Autodesk Inventor part; units mm, degrees
ref_plane "YZ Plane" through (0, 0, 0) normal (1, 0, 0) x (0, 1, 0)
ref_plane "XZ Plane" through (0, 0, 0) normal (0, 1, 0) x (-1, 0, 0)
ref_plane "XY Plane" through (0, 0, 0) normal (0, 0, 1) x (1, 0, 0)
sketch "Sketch1" plane through (0, 0, 0) normal (0, 1, 0) x (-1, 0, 0)
  line L0 (275, 225) -> (-275, 225)
  line L1 (-275, 225) -> (-275, -225)
  line L2 (-275, -225) -> (275, -225)
  line L3 (275, -225) -> (275, 225)
  line L4 (275, 225) -> (-275, -225) construction
  line L5 (-275, 225) -> (275, -225) construction
  point P0 (0, 0)
  dimension "d0" = 550
  dimension "d1" = 450
extrude "Extrusion1" add sketch "Sketch1" against normal blind 15
sketch "Sketch2" plane through (0, -15, 0) normal (0, -1, 0) x (1, 0, 0)
  line L0 (275, -225) -> (275, 225)
  line L1 (275, 225) -> (225, 225)
  line L2 (225, 225) -> (225, 175)
  line L3 (225, 175) -> (275, 175)
  line L4 (275, 175) -> (275, 225)
  line L5 (-275, -225) -> (275, -225)
  line L6 (275, -225) -> (225, -225)
  line L7 (225, -225) -> (225, -175)
  line L8 (225, -175) -> (275, -175)
  line L9 (275, -175) -> (275, -225)
  line L10 (-275, 225) -> (-275, -225)
  line L11 (-275, -225) -> (-225, -225)
  line L12 (-225, -225) -> (-225, -175)
  line L13 (-225, -175) -> (-275, -175)
  line L14 (-275, -175) -> (-275, -225)
  line L15 (-275, 225) -> (-225, 225)
  line L16 (-225, 225) -> (-225, 175)
  line L17 (-225, 175) -> (-275, 175)
  line L18 (-275, 175) -> (-275, 225)
  point P0 (0, 0)
  dimension "d4" = 50
  dimension "d5" = 50
  dimension "d6" = 50
  dimension "d7" = 50
extrude "Extrusion2" add sketch "Sketch2" along normal blind 500
sketch "Sketch3" plane through (0, -515, 0) normal (0, -1, 0) x (1, 0, 0)
  line L0 (225, 175) -> (275, 175)
  line L1 (225, 175) -> (265, 175)
  line L2 (265, 175) -> (265, 215)
  line L3 (265, 215) -> (225, 215)
  line L4 (225, 215) -> (225, 175)
  point P0 (0, 0)
  dimension "d10" = 40
  dimension "d11" = 40
extrude "Extrusion3" cut sketch "Sketch3" against normal blind 500
mirror "Mirror1" about plane through (0, 0, 0) normal (1, 0, 0) of "Extrusion3"
mirror "Mirror2" about plane through (0, 0, 0) normal (0, 0, 1) of "Extrusion3"
sketch "Sketch4" plane through (0, -515, 0) normal (0, -1, 0) x (1, 0, 0)
  line L0 (-275, -175) -> (-225, -175)
  line L1 (-225, -175) -> (-265, -175)
  line L2 (-265, -175) -> (-265, -215)
  line L3 (-265, -215) -> (-225, -215)
  line L4 (-225, -215) -> (-225, -175)
  point P0 (0, 0)
  dimension "d14" = 40
  dimension "d15" = 40
extrude "Extrusion4" cut sketch "Sketch4" against normal blind 500
sketch "Sketch5" plane through (0, 0, 0) normal (0, 1, 0) x (1, 0, 0)
  line L0 (275, -225) -> (275, 225)
  line L1 (275, 0) -> (265, 0)
  line L2 (265, 0) -> (265, -19.5)
  line L3 (265, -19.5) -> (265, 9.5)
  circle A0 centre (265, 9.5) radius 2.5
  circle A1 centre (265, -19.5) radius 2.5
  point P0 (0, 0)
  dimension "d18" = 10
  dimension "d19" = 19.5
  dimension "d20" = 29
  dimension "d21" = 5
  dimension "d22" = 5
extrude "Extrusion5" cut sketch "Sketch5" against normal through all
thread "Thread1"
thread "Thread2"
ref_plane "Work Plane1" through (0, 0, 0) normal (1, 0, 0) x (0, 1, 0)
ref_plane "Work Plane2" through (0, 0, 0) normal (0, 0, 1) x (1, 0, 0)
properties part number "Work table" material "Steel, Mild"
CAD build for the part. Positions are in the model's coordinates, mm. A direction names the side the tool comes from. Round coordinates to 2 decimals unless told otherwise and drop trailing zeros. Order: outer loops, then holes, each group sorted by start corner. A loop starts at its lowest first (then second) coordinate and runs counter-clockwise, first axis right, second up. Notation, with made-up numbers: (86.5, 2.25) -> (104.5, 2.25) arc R26 cw to (104.5, 38.25) -> close; hole circle Ø5 at (-19, 34.5). An arc over 180 degrees is marked (long way). Write item = value, one per line. Start each with the question number.
(1) Pin check, flat tip, straight feed: P1, Ø12, axis at x = 158.5, z = -90, coming from the +Y side. Stop position of the tip, or through.
(2) Cut at C-C, the plane z = 62. List the corners of the cut face in (x, y), then the cut area to 3 significant figures.
(3) Cut at B-B, the plane x = -238.5. List the corners of the cut face in (y, z), then the cut area to 4 significant figures.
(4) Which spindle directions (+Z, -Z, +X, -X, +Y, -Y) get a long thin tool onto all of the face, cutting with end or side? Do faces 4 (the flat face through (265, -268, -195)), 5 (the flat face through (-225.4, -237.2, 225)). Say none if no direction does.
(5) Cut at D-D, the plane x = 169.5. List the corners of the cut face in (y, z), then the cut area to 3 significant figures.
(6) Cut at A-A, the plane y = -128. List the corners of the cut face in (x, z).
(7) Probe line 1 (Z direction, x = 265, y = -6); line 2 (X direction, y = -151.5, z = -178.5); line 3 (Z direction, x = 232, y = -226.5). List the from-to ranges inside material, lowest first. Write a range as [from, to].
(8) Pull direction X, two halves, no side cores. Call faces 1 (the flat face through (275, -218, 184)), 2 (the flat face through (-265, -268, 195)), 3 (the flat face through (266, -515, 211)): released by +X, released by -X, zero draft, split by the parting line, or undercut.
Model answer:
q1.P1 = 0
q2.outline = (-275, -15) -> (275, -15) -> (275, 0) -> (-275, 0) -> close
q2.area = 8,250 mm2
q3.outline = (-515, -225) -> (0, -225) -> (0, 225) -> (-515, 225) -> (-515, 215) -> (-15, 215) -> (-15, -215) -> (-515, -215) -> close
q3.area = 16,750 mm2
q4.face_4 = -Y
q4.face_5 = +Z, +X, -X, +Y, -Y
q5.outline = (-15, -225) -> (0, -225) -> (0, 225) -> (-15, 225) -> close
q5.area = 6,750 mm2
q6.outline = (-275, -225) -> (-225, -225) -> (-225, -215) -> (-265, -215) -> (-265, -175) -> (-275, -175) -> close; (-275, 175) -> (-265, 175) -> (-265, 215) -> (-225, 215) -> (-225, 225) -> (-275, 225) -> close; (225, -225) -> (275, -225) -> (275, -175) -> (265, -175) -> (265, -215) -> (225, -215) -> close; (225, 215) -> (265, 215) -> (265, 175) -> (275, 175) -> (275, 225) -> (225, 225) -> close
q7.line_1 = [-225, -12], [-7, 17], [22, 225]
q7.line_2 = [-275, -265], [265, 275]
q7.line_3 = [-225, -215], [215, 225]
q8.face_1 = released by +X
q8.face_2 = undercut
q8.face_3 = zero draft
